The listing builds one solid part. Answer for the finished solid, in the listing's coordinates (mm). A direction names the side the tool comes from. Round coordinates to 2 decimals unless told otherwise and drop trailing zeros. Loops run counter-clockwise (first coordinate to the right, second up) from the corner with the lowest first, then second, coordinate; pieces in that order, holes last. Notation, with made-up numbers: (-39, 10.5) - (15, 10.5) arc R24 cw to (15, 25.5) - close; hole circle Ø6 at (6, 10.25). An arc over 180 degrees is marked (long way). One line per item, written item: value.
Autodesk Inventor part; units mm, degrees
ref_plane "YZ Plane" through (0, 0, 0) normal (1, 0, 0) x (0, 1, 0)
ref_plane "XZ Plane" through (0, 0, 0) normal (0, 1, 0) x (-1, 0, 0)
ref_plane "XY Plane" through (0, 0, 0) normal (0, 0, 1) x (1, 0, 0)
sketch "Sketch1" plane through (0, 0, 0) normal (0, 0, 1) x (1, 0, 0)
  circle A0 centre (0, 0) radius 3.175
  circle A1 centre (0, 0) radius 1.5875
  line L0 (0, -3.175) -> (19.05, -3.175)
  line L1 (19.05, -3.175) -> (19.05, 0)
  line L2 (19.05, 0) -> (1.5875, 0)
  line L3 (0, -1.5875) -> (0, -3.175)
  dimension "d1" = 6.35
  dimension "d0" = 3.175
  dimension "d2" = 3.175
  dimension "d3" = 19.05
extrude "Extrusion1" add sketch "Sketch1" along normal blind 25.4 contours L2 A1 L3 A0 | L2 L1 L0 A0 | A0 L3 A1 L2
sketch "Sketch2" plane through (0, -3.175, 0) normal (0, -1, 0) x (1, 0, 0)
  line L0 (19.05, 25.4) -> (0, 25.4)
  line L1 (0, 0) -> (19.05, 0)
  line L2 (3.175, 9.525) -> (-3.175, 9.525)
  line L3 (-3.175, 9.525) -> (-3.175, 15.875)
  line L4 (-3.175, 15.875) -> (3.175, 15.875)
  line L5 (3.175, 15.875) -> (3.175, 9.525)
  line L6 (-1.5875, 25.4) -> (1.5875, 25.4)
  line L7 (-3.175, 9.525) -> (3.175, 9.525)
  line L8 (3.175, 9.525) -> (3.175, 0)
  line L9 (3.175, 0) -> (-3.175, 0)
  line L10 (-3.175, 0) -> (-3.175, 9.525)
  line L11 (-3.175, 15.875) -> (3.175, 15.875)
  line L12 (3.175, 15.875) -> (3.175, 25.4)
  line L13 (3.175, 25.4) -> (-3.175, 25.4)
  line L14 (-3.175, 25.4) -> (-3.175, 15.875)
  line L15 (3.175, 9.525) -> (3.175, 0)
  line L16 (0, 0) -> (3.175, 0)
  circle A0 centre (12.7, 19.05) radius 1.5875
  circle A1 centre (12.7, 6.35) radius 1.5875
  dimension "d6" = 6.35
  dimension "d7" = 6.35
  dimension "d8" = 9.525
  dimension "d9" = 3.175
  dimension "d10" = 3.175
  dimension "d13" = 3.175
  dimension "d14" = 3.175
  dimension "d15" = 6.35
  dimension "d16" = 6.35
  dimension "d17" = 12.7
  dimension "d18" = 6.35
extrude "Extrusion2" cut sketch "Sketch2" against normal blind 25.4 contours L12 L4 L14 L13 L6 L0 | L8 L1 L9 L10 L2 | A0 | A1
properties part number "hinge one prong"
1) A cutting plane is placed at B-B on y = -1.25. Give the number of separate pieces and of enclosed holes in the cut face, and give its area (3 significant figures).
Final values:
separate pieces: 2
enclosed holes: 2
area: 414 mm2
2) For a pull along Y with two mould halves and no side action, classify faces 5 (the cylindrical face through (-2.32, 2.17, 12.66)), 6 (the cylindrical face through (-0.34, 1.55, 12.66)), 7 (the flat face through (1.4, -1.5, 15.875)) as released by +Y, released by -Y, zero draft, split by the parting line, or undercut.
Final values:
face 5: split by the parting line
face 6: undercut
face 7: zero draft
3) Consider L1, parallel to Z at x = 12.7, y = -1; L2, parallel to Y at x = 0, z = 14.25 (1 decimal); L3, parallel to Y at x = 5, z = 16 (3 decimals). Determine where each line is inside the solid, lowest interval first.
Final values:
L1: 0 to 4.76, 7.94 to 17.46, 20.64 to 25.4
L2: -3.2 to -1.6, 1.6 to 3.2
L3: -3.175 to 0
4) A cutting plane is placed at A-A on x = 12.7. Give the vertices of the cut face in (y, z) (1 decimal).
Final values:
outline: (-3.2, 0) - (0, 0) - (0, 4.8) - (-3.2, 4.8) - close; (-3.2, 7.9) - (0, 7.9) - (0, 17.5) - (-3.2, 17.5) - close; (-3.2, 20.6) - (0, 20.6) - (0, 25.4) - (-3.2, 25.4) - close
5) Each of these flat-tipped pins is pushed along its axis until it touches: pin 1 Ø3.5 at (x, z) = (12.7, 19.05) entering from -Y (3 decimals); pin 2 Ø3 at (x, y) = (1.5, -1) entering from +Z (3 decimals); pin 3 Ø5 at (x, z) = (8.5, 14) entering from +Y; pin 4 Ø1.6 at (y, z) = (-1, 3) entering from -X (3 decimals). Where does it stop, or does it pass through?
Final values:
pin 1: y = -3.175
pin 2: z = 15.875
pin 3: y = 0
pin 4: x = 3.175
6) For faces 1 (the flat face through (3.175, -2, 21)), 2 (the flat face through (11, -2, 25.4)), 3 (the flat face through (11, 0, 13)), 4 (the flat face through (3.175, -2, 5)), determine the directions among +Z, -Z, +X, -X, +Y, -Y from which every point of the face is accessible in a straight line to the end or side of a thin tool.
Final values:
face 1: +Z, -X, +Y, -Y
face 2: +Z, +X, -X, +Y, -Y
face 3: +Z, -Z, +X, +Y
face 4: -Z, -X, +Y, -Y
7) A cutting plane is placed at D-D on y = 1.25. Give the vertices of the cut face in (x, z) (3 decimals).
Final values:
outline: (-2.919, 9.525) - (-0.979, 9.525) - (-0.979, 15.875) - (-2.919, 15.875) - close; (0.979, 9.525) - (2.919, 9.525) - (2.919, 15.875) - (0.979, 15.875) - close
